Verification items for the finished model (mm, model axes). Give positions to 0.01 mm unless a question says otherwise; leave off trailing zeros. Answer in a Markdown table with one row per item.
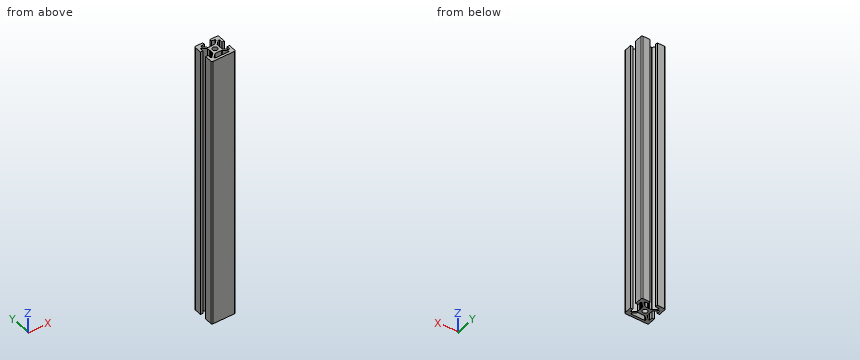
Autodesk Inventor part; units mm, degrees
ref_plane "C1_XY" through (0, 0, 0) normal (0, 0, 1) x (1, 0, 0)
ref_plane "C1_YZ" through (0, 0, 0) normal (1, 0, 0) x (0, 1, 0)
ref_plane "C1_ZX" through (0, 0, 0) normal (0, 1, 0) x (0, 0, 1)
sketch "Sketch_76" plane through (0, 0, 0) normal (0, 0, 1) x (1, 0, 0)
  line L0 (-10, -3) -> (-10, -9)
  arc A0 (-10, -9) -> (-9, -10) centre (-9, -9) ccw
  line L1 (-9, -10) -> (9, -10)
  arc A1 (9, -10) -> (10, -9) centre (9, -9) ccw
  line L2 (10, -9) -> (10, -3)
  line L3 (10, -3) -> (8, -3)
  line L4 (8, -3) -> (8, -6)
  line L5 (8, -6) -> (7.0607, -6)
  line L6 (7.0607, -6) -> (4, -2.9393)
  line L7 (4, -2.9393) -> (4, -0.6536)
  arc A2 (4, -0.6536) -> (3.933, -0.4036) centre (3.5, -0.6536) ccw
  line L8 (3.933, -0.4036) -> (3.7, 0)
  line L9 (3.7, 0) -> (3.933, 0.4036)
  arc A3 (3.933, 0.4036) -> (3.933, 0.9036) centre (3.5, 0.6536) ccw
  line L10 (3.933, 0.9036) -> (3.751, 1.2189)
  line L11 (3.751, 1.2189) -> (4, 2.5)
  line L12 (4, 2.5) -> (4, 2.9393)
  line L13 (4, 2.9393) -> (7.0607, 6)
  line L14 (7.0607, 6) -> (8, 6)
  line L15 (8, 6) -> (8, 3)
  line L16 (8, 3) -> (10, 3)
  line L17 (10, 3) -> (10, 9)
  arc A4 (10, 9) -> (9, 10) centre (9, 9) ccw
  line L18 (9, 10) -> (3, 10)
  line L19 (3, 10) -> (3, 8)
  line L20 (3, 8) -> (6, 8)
  line L21 (6, 8) -> (6, 7.0607)
  line L22 (6, 7.0607) -> (2.9393, 4)
  line L23 (2.9393, 4) -> (0.6536, 4)
  arc A5 (0.6536, 4) -> (0.4036, 3.933) centre (0.6536, 3.5) ccw
  line L24 (0.4036, 3.933) -> (0, 3.7)
  line L25 (0, 3.7) -> (-0.4036, 3.933)
  arc A6 (-0.4036, 3.933) -> (-0.9036, 3.933) centre (-0.6536, 3.5) ccw
  line L26 (-0.9036, 3.933) -> (-1.2189, 3.751)
  line L27 (-1.2189, 3.751) -> (-2.5, 4)
  line L28 (-2.5, 4) -> (-2.9393, 4)
  line L29 (-2.9393, 4) -> (-6, 7.0607)
  line L30 (-6, 7.0607) -> (-6, 8)
  line L31 (-6, 8) -> (-3, 8)
  line L32 (-3, 8) -> (-3, 10)
  line L33 (-3, 10) -> (-9, 10)
  arc A7 (-9, 10) -> (-10, 9) centre (-9, 9) ccw
  line L34 (-10, 9) -> (-10, 3)
  line L35 (-10, 3) -> (-8, 3)
  line L36 (-8, 3) -> (-8, 6)
  line L37 (-8, 6) -> (-7.0607, 6)
  line L38 (-7.0607, 6) -> (-4, 2.9393)
  line L39 (-4, 2.9393) -> (-4, 0.6536)
  arc A8 (-4, 0.6536) -> (-3.933, 0.4036) centre (-3.5, 0.6536) ccw
  line L40 (-3.933, 0.4036) -> (-3.7, 0)
  line L41 (-3.7, 0) -> (-3.933, -0.4036)
  arc A9 (-3.933, -0.4036) -> (-3.933, -0.9036) centre (-3.5, -0.6536) ccw
  line L42 (-3.933, -0.9036) -> (-3.751, -1.2189)
  line L43 (-3.751, -1.2189) -> (-4, -2.5)
  line L44 (-4, -2.5) -> (-4, -2.9393)
  line L45 (-4, -2.9393) -> (-7.0607, -6)
  line L46 (-7.0607, -6) -> (-8, -6)
  line L47 (-8, -6) -> (-8, -3)
  line L48 (-8, -3) -> (-10, -3)
  line L49 (-6, -7.2678) -> (-6, -7.5)
  arc A10 (-6, -7.5) -> (-5.5, -8) centre (-5.5, -7.5) ccw
  line L50 (-5.5, -8) -> (5.5, -8)
  arc A11 (5.5, -8) -> (6, -7.5) centre (5.5, -7.5) ccw
  line L51 (6, -7.5) -> (6, -7.2678)
  arc A12 (6, -7.2678) -> (5.8536, -6.9142) centre (5.5, -7.2678) ccw
  line L52 (5.8536, -6.9142) -> (3.0858, -4.1464)
  arc A13 (3.0858, -4.1464) -> (2.7322, -4) centre (2.7322, -4.5) ccw
  line L53 (2.7322, -4) -> (-2.7322, -4)
  arc A14 (-2.7322, -4) -> (-3.0858, -4.1464) centre (-2.7322, -4.5) ccw
  line L54 (-3.0858, -4.1464) -> (-5.8536, -6.9142)
  arc A15 (-5.8536, -6.9142) -> (-6, -7.2678) centre (-5.5, -7.2678) ccw
extrude "Extrusion1" add sketch "Sketch_76" against normal blind 231
sketch "Sketch2" plane through (0, 0, -231) normal (0, 0, -1) x (-1, 0, 0)
  point P0 (0, 0)
hole "Hole1" at (0, 0, -231) direction (0, 0, 1) diameter 4.2 depth 231
ref_plane "C1_XY" through (0, 0, 0) normal (0, 0, 1) x (1, 0, 0)
ref_plane "C1_YZ" through (0, 0, 0) normal (1, 0, 0) x (0, 1, 0)
ref_plane "C1_ZX" through (0, 0, 0) normal (0, 1, 0) x (0, 0, 1)
properties part number "NFSF5-2020-231"
Item 1: Go/stop test with a flat-tipped pin: pin 1 (0.7 mm diameter, centred on y = 2, z = -84.5, fed in from -X). Record where the tip stops, or that it passes through.
Reported:
| item | result |
|---|---|
| pin 1 | stops at x = -4 |
Item 2: Sectioned sample at A-A (z = -17). State how many separate pieces and enclosed holes the cut face has, and give its area (3 significant figures).
Reported:
| item | result |
|---|---|
| separate pieces | 1 |
| enclosed holes | 2 |
| area | 194 mm^2 |
Item 3: Scan lines: L1, parallel to Y at x = 0, z = -126.5; L2, parallel to X at y = 4.75, z = -37.5; L3, parallel to X at y = 0, z = -62. Record each from-to range of solid material in increasing order. Write a range as [from, to].
Reported:
| item | result |
|---|---|
| L1 | y = [-10, -8], [-4, -2.1], [2.1, 3.7] |
| L2 | x = [-10, -8], [-5.81, -3.69], [3.69, 5.81], [8, 10] |
| L3 | x = [-3.7, -2.1], [2.1, 3.7] |
